CAD build for the part. Positions are in the model's coordinates, mm. Give positions to 0.01 mm unless a question says otherwise; leave off trailing zeros. Loops run counter-clockwise (first coordinate to the right, second up) from the corner with the lowest first, then second, coordinate; pieces in that order, holes last.
Item 1: Probe probe 1 along X at (y, z) = (100.5, 1.5); probe 2 along X at (y, z) = (101, -2.5); probe 3 along Y at (x, z) = (40.5, -1). List the from-to ranges inside material, lowest first.
Item 2: Saw through at B-B on y = 179. Give the cut face in (x, z) (3 decimals).
Item 3: Saw through at A-A on x = 2. Give the cut face in (y, z) (3 decimals).
Item 4: Drop flat-ended pins along their axis: P1, Ø1, axis at x = -8.5, z = 2, coming from the -Y side; P2, Ø2, axis at x = -32, z = 2, coming from the +Y side; P3, Ø1.9, axis at y = 101, z = 0, coming from the -X side. Give the stop position or say it passes through.
from build123d import *

# Parameters (mm, degrees)
BOSS_EXTRUDE1_DEPTH = 3.175
SKETCH2_W           = 6.35
SKETCH2_H           = 25.4
BOSS_EXTRUDE2_DEPTH = 6.35
LPATTERN1_COUNT     = 3
LPATTERN1_PITCH     = 50.8
SKETCH3_W           = 25.4
SKETCH3_H           = 6.35
BOSS_EXTRUDE3_DEPTH = 6.35
LPATTERN2_COUNT     = 2
LPATTERN2_PITCH     = 50.8
CUT_EXTRUDE1_DEPTH  = 292.166765647


with BuildPart() as part:
    # Sketch1 → Boss-Extrude1 (new, symmetric)
    with BuildSketch(Plane.XY):
        Polygon((49.19007938, 285.75), (49.19007938, 95.25), (-52.40992062, 95.25), align=None)
    extrude(amount=BOSS_EXTRUDE1_DEPTH, both=True)

    # Sketch2 → Boss-Extrude2 (add)
    with BuildSketch(Plane(origin=(49.19007938, 0, 0), x_dir=(0, 0, -1), z_dir=(1, 0, 0))):
        with Locations((0, 133.35)):
            Rectangle(SKETCH2_W, SKETCH2_H)
    boss_extrude2 = extrude(amount=BOSS_EXTRUDE2_DEPTH)

    # LPattern1: Boss-Extrude2 ×3
    with Locations(*[(0, i * LPATTERN1_PITCH, 0) for i in range(1, LPATTERN1_COUNT)]):
        add(boss_extrude2)

    # Sketch3 → Boss-Extrude3 (add)
    with BuildSketch(Plane.XZ.offset(-95.25)):
        with Locations((11.09007938, 0)):
            Rectangle(SKETCH3_W, SKETCH3_H)
    boss_extrude3 = extrude(amount=BOSS_EXTRUDE3_DEPTH)

    # LPattern2: Boss-Extrude3 ×2
    with Locations(*[(-i * LPATTERN2_PITCH, 0, 0) for i in range(1, LPATTERN2_COUNT)]):
        add(boss_extrude3)

    # Sketch4 → Cut-Extrude1 (cut, through all)
    with BuildSketch(Plane.XY.offset(3.175)):
        Polygon((49.19007938, 156.6545), (49.19007938, 160.8455), (40.42707938, 160.8455), (40.42707938, 162.179), (37.88707938, 162.179), (37.88707938, 160.8455), (34.58507938, 160.8455), (34.58507938, 156.6545), (37.88707938, 156.6545), (37.88707938, 155.321), (40.42707938, 155.321), (40.42707938, 156.6545), align=None)
        Polygon((-16.40542062, 95.25), (-12.21442062, 95.25), (-12.21442062, 104.013), (-10.88092062, 104.013), (-10.88092062, 106.553), (-12.21442062, 106.553), (-12.21442062, 109.855), (-16.40542062, 109.855), (-16.40542062, 106.553), (-17.73892062, 106.553), (-17.73892062, 104.013), (-16.40542062, 104.013), align=None)
        Polygon((49.19007938, 207.4545), (49.19007938, 211.6455), (40.42707938, 211.6455), (40.42707938, 212.979), (37.88707938, 212.979), (37.88707938, 211.6455), (34.58507938, 211.6455), (34.58507938, 207.4545), (37.88707938, 207.4545), (37.88707938, 206.121), (40.42707938, 206.121), (40.42707938, 207.4545), align=None)
        Polygon((34.39457938, 95.25), (38.58557938, 95.25), (38.58557938, 104.013), (39.91907938, 104.013), (39.91907938, 106.553), (38.58557938, 106.553), (38.58557938, 109.855), (34.39457938, 109.855), (34.39457938, 106.553), (33.06107938, 106.553), (33.06107938, 104.013), (34.39457938, 104.013), align=None)
    extrude(amount=-CUT_EXTRUDE1_DEPTH, mode=Mode.SUBTRACT)


solid = part.part
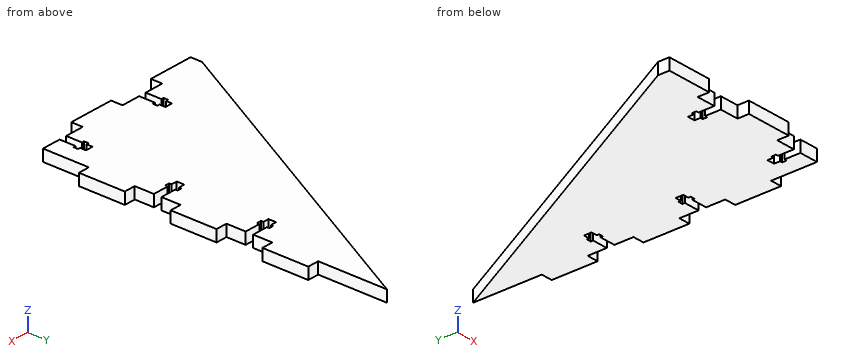
Results below:
1. probe 1: x = -49.61 to -16.41, -12.21 to 34.39, 38.59 to 49.19
1. probe 2: x = -49.34 to -16.41, -12.21 to 34.39, 38.59 to 49.19
1. probe 3: y = 95.25 to 156.65, 160.85 to 207.45, 211.65 to 269.46
2. outline: (-7.743, -3.175) - (55.54, -3.175) - (55.54, 3.175) - (-7.743, 3.175) - close
3. outline: (88.9, -3.175) - (197.269, -3.175) - (197.269, 3.175) - (88.9, 3.175) - close
4. P1: stops at y = 95.25
4. P2: stops at y = 135.39
4. P3: stops at x = -49.85
